For this review, take the finished solid that the model builds, in its own axes (mm). Round coordinates to 2 decimals unless told otherwise and drop trailing zeros. Order: outer loops, then holes, each group sorted by start corner. A loop starts at its lowest first (then second) coordinate and runs counter-clockwise, first axis right, second up. Notation, with made-up numbers: M -35.75,80.5 L -23.75,80.5 A26 cw -23.75,110.5 Z; hole C 28,16.5 d3. An arc over 180 degrees is marked long. Answer as a JSON object with one key per item and string values.
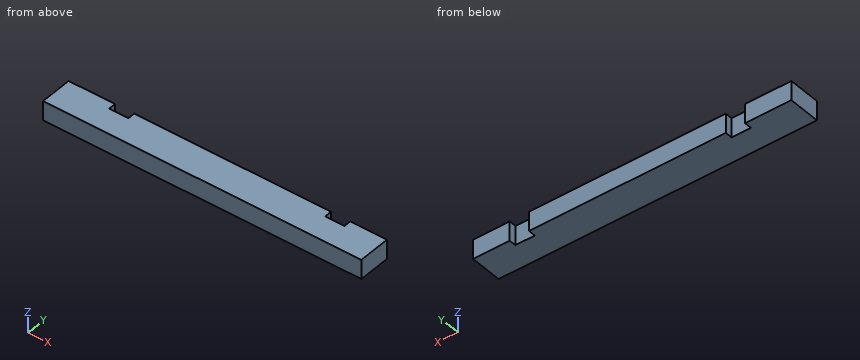
Autodesk Inventor part; units mm, degrees
ref_plane "YZ Plane" through (0, 0, 0) normal (1, 0, 0) x (0, 1, 0)
ref_plane "XZ Plane" through (0, 0, 0) normal (0, 1, 0) x (-1, 0, 0)
ref_plane "XY Plane" through (0, 0, 0) normal (0, 0, 1) x (1, 0, 0)
sketch "Sketch1" plane through (0, 0, 0) normal (0, 0, 1) x (1, 0, 0)
  line L0 (0, 0) -> (0, 42.3672)
  line L1 (0, 42.3672) -> (60.96, 42.3672)
  line L2 (60.96, 42.3672) -> (60.96, 32.8422)
  line L3 (60.96, 32.8422) -> (86.36, 32.8422)
  line L4 (86.36, 32.8422) -> (86.36, 42.3672)
  line L5 (86.36, 42.3672) -> (345.44, 42.3672)
  line L6 (345.44, 42.3672) -> (345.44, 32.8422)
  line L7 (345.44, 32.8422) -> (370.84, 32.8422)
  line L8 (370.84, 32.8422) -> (370.84, 42.3672)
  line L9 (370.84, 42.3672) -> (419.1, 42.3672)
  line L10 (419.1, 42.3672) -> (419.1, 0)
  line L11 (419.1, 0) -> (0, 0)
  dimension "d0" = 42.3672
  dimension "d1" = 60.96
  dimension "d2" = 25.4
  dimension "d3" = 345.44
  dimension "d4" = 419.1
  dimension "d5" = 25.4
  dimension "d6" = 9.525
extrude "Extrusion1" add sketch "Sketch1" against normal blind 25.4
properties part number "mid spacer"
1) Insertion check: P1, Ø7.5, axis at y = 39.5, z = -14, coming from the -X side; P2, Ø7.5, axis at x = 71.5, z = -9.5, coming from the +Y side. Each pin has a flat end and moves straight along its axis. Give the tip position at first contact, or say it passes through.
Geometry check:
{"P1": "stops at x = 0", "P2": "stops at y = 32.84"}
2) Add section A-A on z = -5. State the section outline as (x, y) points.
Geometry check:
{"outline": "M 0,0 L 419.1,0 L 419.1,42.37 L 370.84,42.37 L 370.84,32.84 L 345.44,32.84 L 345.44,42.37 L 86.36,42.37 L 86.36,32.84 L 60.96,32.84 L 60.96,42.37 L 0,42.37 Z"}
3) For L1, parallel to X at y = 34.5, z = -21.75; L2, parallel to Y at x = 64, z = -11, list the stretches that pass through material, from the lowest coordinate up.
Geometry check:
{"L1": "x = 0 to 60.96, 86.36 to 345.44, 370.84 to 419.1", "L2": "y = 0 to 32.84"}
